Input: part model. Units: mm. Frame: model coordinates. A direction names the side the tool comes from. Round coordinates to 2 decimals unless told otherwise and drop trailing zeros. Loops run counter-clockwise (first coordinate to the right, second up) from the corner with the lowest first, then second, coordinate; pieces in that order, holes last.
1) Access query for faces 1 (the face through (0, 46, -2)), 2 (the face through (-18, 29, 19)), 3 (the face through (-18, 9.4, 18)), 4 (the face through (-3.417, 34.986, -0.759)), 5 (the face through (-16, 10, 15)). Directions: +Z, -Z, +X, -X, +Y, -Y. A direction counts if a zero-diameter tool reaches every point of the face in a straight line with its end or side. Return the directions, or none.
2) Section A-A, the plane x = 0. Return loops of the section in (y, z).
3) Section B-B, the plane z = 0. Return loops of the section in (x, y), and give its area (3 significant figures).
4) Draft query along Y for faces 6 (the face through (-16, 10, -16)), 7 (the face through (-14.45, 31.78, -16.64)), 8 (the face through (-18, 24.6, -18)), 9 (the face through (-18, 9.4, -18)). Return one class per face: pulls with the +Y half, pulls with the -Y half, needs draft (parallel to the pull), parting line crosses it, or undercut.
5) First-contact query: pin 1 (3 mm diameter, centred on x = -2, y = 43, fed in from -Z); pin 2 (1.6 mm diameter, centred on x = 15.5, z = 15, fed in from -Y); pin 3 (5.5 mm diameter, centred on x = -19, z = -16.5, fed in from +Y). Flat tips, straight axial feed; report the tip coordinate or a pass-through.
6) Section D-D, the plane x = 10. Return loops of the section in (y, z).
7) Section C-C, the plane y = 47. Return loops of the section in (x, z).
8) Ray query, line 1 along X through (y, z) = (32.1, 15.5); line 2 along Y through (x, z) = (-17, -19); line 3 along Y through (x, z) = (4, 12.5). Return the intervals inside material, ascending.
from build123d import *

# Parameters (mm, degrees)
SKETCH4_W               = 42
SKETCH4_H               = 42
BOTTOM_DEPTH            = 9.4
MIDDLE_DEPTH            = 15.2
SKETCH8_W               = 42
SKETCH8_H               = 42
TOP_DEPTH               = 9.4
CHAMFER1_SIZE           = 5
SKETCH9_R               = 11
SKETCH9_R_2             = 3.5
RING_DEPTH              = 2
SKETCH10_R              = 2.5
SHAFT_DEPTH             = 20
SKETCH12_R              = 1.55
CUT_EXTRUDE4_DEPTH      = 4.5
CUT_EXTRUDE5_START      = -10
SKETCH15_R              = 1.55
CUT_EXTRUDE5_DEPTH      = 10
BOSS_EXTRUDE1_START     = 10
SKETCH16_R              = 2.5
BOSS_EXTRUDE1_DEPTH     = 10
CUT_EXTRUDE3_DEPTH      = 5
CUT_EXTRUDE3_DEPTH_BACK = 5
SKETCH11_W              = 1.458446266
SKETCH11_H              = 24.242457261
SKETCH11_W_2            = 8.851647276
SKETCH11_H_2            = 12.03282496


with BuildPart() as part:
    # Sketch4 → Bottom (new body)
    with BuildSketch(Plane(origin=(0, 0, 0), x_dir=(1, 0, 0), z_dir=(0, 1, 0))):
        Rectangle(SKETCH4_W, SKETCH4_H)
    extrude(amount=BOTTOM_DEPTH)

    # Sketch6 → Middle (add)
    with BuildSketch(Plane(origin=(0, 9.4, 0), x_dir=(1, 0, 0), z_dir=(0, 1, 0))):
        Polygon((-21, -14), (-14, -21), (14, -21), (21, -14), (21, 14), (14, 21), (-14, 21), (-21, 14), align=None)
    extrude(amount=MIDDLE_DEPTH)

    # Sketch8 → Top (add)
    with BuildSketch(Plane(origin=(0, 24.6, 0), x_dir=(1, 0, 0), z_dir=(0, 1, 0))):
        Rectangle(SKETCH8_W, SKETCH8_H)
    extrude(amount=TOP_DEPTH)

    # Chamfer1
    chamfer1_edges = [part.edges().sort_by_distance(p)[0] for p in [
        (21, 29.3, 21),
        (21, 29.3, -21),
        (-21, 29.3, -21),
        (-21, 29.3, 21),
        (-21, 4.7, 21),
        (-21, 4.7, -21),
        (21, 4.7, -21),
        (21, 4.7, 21),
    ]]
    chamfer(chamfer1_edges, length=CHAMFER1_SIZE)

    # Sketch9 → Ring (add)
    with BuildSketch(Plane(origin=(0, 34, 0), x_dir=(1, 0, 0), z_dir=(0, 1, 0))):
        with Locations(Location((0, 0, 0), (0, 0, 270))):
            Circle(SKETCH9_R)
        with Locations(Location((0, 0, 0), (0, 0, 270))):
            Circle(SKETCH9_R_2, mode=Mode.SUBTRACT)
    extrude(amount=RING_DEPTH)

    # Sketch10 → Shaft (add)
    with BuildSketch(Plane(origin=(0, 34, 0), x_dir=(1, 0, 0), z_dir=(0, 1, 0))):
        with Locations(Location((0, 0, 0), (0, 0, 90))):
            Circle(SKETCH10_R)
    extrude(amount=SHAFT_DEPTH)

    # Sketch12 → Cut-Extrude4 (cut)
    with BuildSketch(Plane(origin=(0, 34, 0), x_dir=(1, 0, 0), z_dir=(0, 1, 0))):
        with Locations(Location((15.5, -15.5, 0), (0, 0, 270))):
            Circle(SKETCH12_R)
        with Locations(Location((-15.5, -15.5, 0), (0, 0, 270))):
            Circle(SKETCH12_R)
        with Locations(Location((-15.5, 15.5, 0), (0, 0, 270))):
            Circle(SKETCH12_R)
        with Locations(Location((15.5, 15.5, 0), (0, 0, 270))):
            Circle(SKETCH12_R)
    extrude(amount=-CUT_EXTRUDE4_DEPTH, mode=Mode.SUBTRACT)

    # Sketch15 → Cut-Extrude5 (cut)
    with BuildSketch(Plane.XZ.offset(CUT_EXTRUDE5_START)):
        with Locations(Location((15.5, 15.5, 0), (0, 0, 90))):
            Circle(SKETCH15_R)
        with Locations(Location((15.5, -15.5, 0), (0, 0, 90))):
            Circle(SKETCH15_R)
        with Locations(Location((-15.5, 15.5, 0), (0, 0, 90))):
            Circle(SKETCH15_R)
        with Locations(Location((-15.5, -15.5, 0), (0, 0, 90))):
            Circle(SKETCH15_R)
    extrude(amount=CUT_EXTRUDE5_DEPTH, mode=Mode.SUBTRACT)

    # Sketch16 → Boss-Extrude1 (add)
    with BuildSketch(Plane(origin=(0, 0, 0), x_dir=(-1, 0, 0), z_dir=(0, -1, 0)).offset(BOSS_EXTRUDE1_START)):
        with Locations(Location((0, 0, 0), (0, 0, 90))):
            Circle(SKETCH16_R)
    extrude(amount=-BOSS_EXTRUDE1_DEPTH)

    # Sketch11 → Cut-Extrude3 (cut, two sides: drawn at the far end of the back side and taken through both)
    with BuildSketch(Plane(origin=(0, 0, 0), x_dir=(0, 0, -1), z_dir=(1, 0, 0)).offset(-CUT_EXTRUDE3_DEPTH_BACK)):
        with Locations((2.729223133, 51.12122863)):
            Rectangle(SKETCH11_W, SKETCH11_H)
        with Locations((6.425823638, -7.01641248)):
            Rectangle(SKETCH11_W_2, SKETCH11_H_2)
    extrude(amount=CUT_EXTRUDE3_DEPTH + CUT_EXTRUDE3_DEPTH_BACK, mode=Mode.SUBTRACT)


solid = part.part
Final values:
1. face 1: -Z, +X, -X, +Y
1. face 2: +Z, -X, +Y, -Y
1. face 3: +Z, -X
1. face 4: +Y
1. face 5: -Y
2. outline: (-10, -2) - (-1, -2) - (-1, -2.5) - (0, -2.5) - (0, -21) - (34, -21) - (34, -11) - (36, -11) - (36, -3.5) - (34, -3.5) - (34, -2.5) - (39, -2.5) - (39, -2) - (54, -2) - (54, 2.5) - (34, 2.5) - (34, 3.5) - (36, 3.5) - (36, 11) - (34, 11) - (34, 21) - (0, 21) - (0, 2.5) - (-10, 2.5) - close
3. outline: (-21, 0) - (-2.5, 0) - (-2.5, -10) - (2.5, -10) - (2.5, 0) - (21, 0) - (21, 34) - (11, 34) - (11, 36) - (3.5, 36) - (3.5, 34) - (2.5, 34) - (2.5, 54) - (-2.5, 54) - (-2.5, 34) - (-3.5, 34) - (-3.5, 36) - (-11, 36) - (-11, 34) - (-21, 34) - close
3. area: 1,610 mm2
4. face 6: pulls with the -Y half
4. face 7: needs draft
4. face 8: undercut
4. face 9: undercut
5. pin 1: stops at z = -2
5. pin 2: stops at y = 10
5. pin 3: stops at y = 34
6. outline: (0, -21) - (34, -21) - (34, -4.58) - (36, -4.58) - (36, 4.58) - (34, 4.58) - (34, 21) - (0, 21) - close
7. outline: (-1.5, -2) - (1.5, -2) arc R2.5 ccw (long way) to start
8. line 1: x = -21 to -17.05, -13.95 to 13.95, 17.05 to 21
8. line 2: y = 0 to 9.4, 24.6 to 34
8. line 3: y = 0 to 34
